Autodesk Inventor part; units mm, degrees
ref_plane "YZ Plane" through (0, 0, 0) normal (1, 0, 0) x (0, 1, 0)
ref_plane "XZ Plane" through (0, 0, 0) normal (0, 1, 0) x (-1, 0, 0)
ref_plane "XY Plane" through (0, 0, 0) normal (0, 0, 1) x (1, 0, 0)
sketch "Sketch6" plane through (0, 0, 0) normal (0, 1, 0) x (-1, 0, 0)
  line L0 (255.9, -490) -> (-255.9, -490)
  line L1 (-255.9, -490) -> (-255.9, 490)
  line L2 (-255.9, 490) -> (255.9, 490)
  line L3 (255.9, 490) -> (255.9, -490)
  line L4 (255.9, -490) -> (-255.9, 490) construction
  line L5 (-255.9, -490) -> (255.9, 490) construction
  point P0 (0, 0)
  dimension "d52" = 511.8
  dimension "d53" = 980
extrude "Plate2" add sketch "Sketch6" along normal blind 0.5
sketch "Sketch11" plane through (-255.4, 0, 490) normal (-1, 0, 0) x (0, -1, 0)
  line L0 (0, -980) -> (0, 0)
  line L1 (0, 0) -> (-10, 0)
  line L2 (-10, 0) -> (-10, -980)
  line L3 (-10, -980) -> (0, -980)
edge flange "Flange2" height 10 angle 90 thickness 0.5 bend radius 0.5 thickness toward (-1, 0, 0) relief tear relief width 0.5 relief depth 0.25 edges at (-255.9, 0.5, 0) wall of the first edge with corners at (-255.4, 0, -490) (-255.4, 0, 490) (-255.4, 10, 490) (-255.4, 10, -490)
bend "Bend3"
corner "Corner3"
sketch "Sketch12" plane through (-255.9, 9.5, 490) normal (0, 1, 0) x (-1, 0, 0)
  line L0 (0, -980) -> (0, 0)
  line L1 (0, 0) -> (-10, 0)
  line L2 (-10, 0) -> (-10, -980)
  line L3 (-10, -980) -> (0, -980)
edge flange "Flange3" height 10 angle 90 thickness 0.5 bend radius 0.5 thickness toward (0, 1, 0) relief tear relief width 0.5 relief depth 0.25 edges at (-255.4, 10, 0) wall of the first edge with corners at (-255.9, 9.5, -490) (-255.9, 9.5, 490) (-245.9, 9.5, 490) (-245.9, 9.5, -490)
bend "Bend4"
corner "Corner4"
sketch "Sketch13" plane through (255.4, 0, -490) normal (1, 0, 0) x (0, 1, 0)
  line L0 (0, 980) -> (0, 0)
  line L1 (0, 0) -> (10, 0)
  line L2 (10, 0) -> (10, 980)
  line L3 (10, 980) -> (0, 980)
edge flange "Flange4" height 10 angle 90 thickness 0.5 bend radius 0.5 thickness toward (1, 0, 0) relief tear relief width 0.5 relief depth 0.25 edges at (255.9, 0.5, 0) wall of the first edge with corners at (255.4, 0, 490) (255.4, 0, -490) (255.4, 10, -490) (255.4, 10, 490)
bend "Bend5"
corner "Corner5"
sketch "Sketch14" plane through (255.9, 9.5, -490) normal (0, 1, 0) x (-1, 0, 0)
  line L0 (0, 980) -> (0, 0)
  line L1 (0, 0) -> (10, 0)
  line L2 (10, 0) -> (10, 980)
  line L3 (10, 980) -> (0, 980)
edge flange "Flange5" height 10 angle 90 thickness 0.5 bend radius 0.5 thickness toward (0, 1, 0) relief tear relief width 0.5 relief depth 0.25 edges at (255.4, 10, 0) wall of the first edge with corners at (255.9, 9.5, 490) (255.9, 9.5, -490) (245.9, 9.5, -490) (245.9, 9.5, 490)
bend "Bend6"
corner "Corner6"
fillet "Corner Round1" radius 4 4 edges at (245.9, 9.75, -490) (-245.9, 9.75, -490) (-245.9, 9.75, 490) (245.9, 9.75, 490)
equation "\"d52\" = ЖАБРЫ_базовая_ширина - 4 * ЖАБРЫ_шаг_листов"
equation "\"d53\" = ЖАБРЫ_базовая_длина_кор_лист"
equation "\"d54\" = Thickness"
equation "\"d84\" = BendReliefWidth"
equation "\"d85\" = BendReliefDepth"
equation "\"d86\" = MinimumRemnant"
equation "\"d87\" = TransitionRadius"
equation "\"d90\" = BendRadius"
equation "\"d91\" = CornerReliefSize"
equation "\"d92\" = GapSize"
equation "\"d93\" = JacobiRadiusSize"
equation "\"d94\" = BendReliefWidth"
equation "\"d95\" = BendReliefDepth"
equation "\"d96\" = MinimumRemnant"
equation "\"d97\" = TransitionRadius"
equation "\"d100\" = BendRadius"
equation "\"d101\" = CornerReliefSize"
equation "\"d102\" = GapSize"
equation "\"d103\" = JacobiRadiusSize"
equation "\"d104\" = BendReliefWidth"
equation "\"d105\" = BendReliefDepth"
equation "\"d106\" = MinimumRemnant"
equation "\"d107\" = TransitionRadius"
equation "\"d110\" = BendRadius"
equation "\"d111\" = CornerReliefSize"
equation "\"d112\" = GapSize"
equation "\"d113\" = JacobiRadiusSize"
equation "\"d114\" = BendReliefWidth"
equation "\"d115\" = BendReliefDepth"
equation "\"d116\" = MinimumRemnant"
equation "\"d117\" = TransitionRadius"
equation "\"d120\" = BendRadius"
equation "\"d121\" = CornerReliefSize"
equation "\"d122\" = GapSize"
equation "\"d123\" = JacobiRadiusSize"
equation "\"BendRadius\" = Thickness"
equation "\"BendReliefWidth\" = Thickness"
equation "\"BendReliefDepth\" = 0.5 * Thickness"
equation "\"CornerReliefSize\" = 4 * Thickness"
equation "\"MinimumRemnant\" = 2 * Thickness"
equation "\"TransitionRadius\" = BendRadius"
equation "\"JacobiRadiusSize\" = BendRadius"
equation "\"GapSize\" = Thickness"
properties part number "MSC 808 SHEET GILLS" material "Stainless Steel"
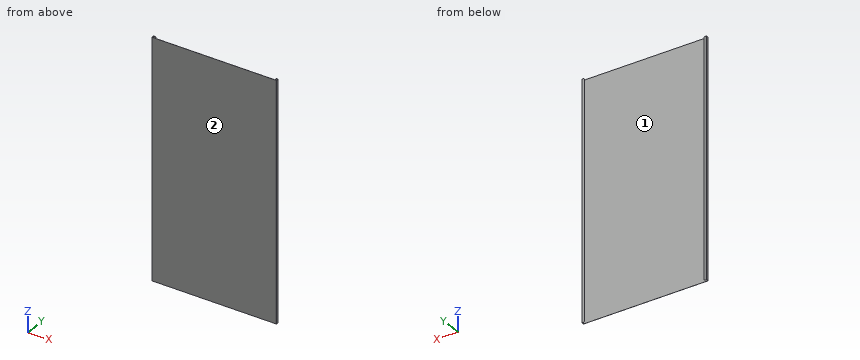
For this review, take the finished solid that the model builds, in its own axes (mm). Face numbers are marked on the shaded views. Round coordinates to 2 decimals unless told otherwise and drop trailing zeros. Loops run counter-clockwise (first coordinate to the right, second up) from the corner with the lowest first, then second, coordinate; pieces in that order, holes last.
Q1. Insertion check: pin 1 Ø0.6 at (y, z) = (9.5, -242) entering from +X; pin 2 Ø8 at (x, z) = (127.5, -306) entering from +Y. Each pin has a flat end and moves straight along its axis. Give the tip position at first contact, or say it passes through.
Result sheet:
pin 1: stops at x = 255.88
pin 2: stops at y = 0.5
Q2. To check wall thickness, follow line 1 along X through (y, z) = (4.75, -88.5); line 2 along Y through (x, z) = (187, -203.5). State the ranges of each line that lie inside material, in increasing order.
Result sheet:
line 1: x = -255.9 to -255.4, 255.4 to 255.9
line 2: y = 0 to 0.5
Q3. Add section C-C on x = -216. Write out the cut boundary in (y, z), plus the area to 3 significant figures.
Result sheet:
outline: (0, -490) - (0.5, -490) - (0.5, 490) - (0, 490) - close
area: 490 mm2
Q4. Add section A-A on y = 6.5. Write out the cut boundary in (x, z).
Result sheet:
outline: (-255.9, -490) - (-255.4, -490) - (-255.4, 490) - (-255.9, 490) - close; (255.4, -490) - (255.9, -490) - (255.9, 490) - (255.4, 490) - close
Q5. Mouldability with a two-part tool opening along X and no side actions: class the marked faces 1 and 2 as +X half, -X half, draft (parallel to the pull), parting line (faces both ways), or undercut.
Result sheet:
face 1: undercut
face 2: draft
Q6. Add section B-B on z = -211. Write out the cut boundary in (x, y).
Result sheet:
outline: (-255.9, 1) arc R1 ccw to (-254.9, 0) - (254.9, 0) arc R1 ccw to (255.9, 1) - (255.9, 9) arc R1 ccw to (254.9, 10) - (245.9, 10) - (245.9, 9.5) - (254.9, 9.5) arc R0.5 cw to (255.4, 9) - (255.4, 1) arc R0.5 cw to (254.9, 0.5) - (-254.9, 0.5) arc R0.5 cw to (-255.4, 1) - (-255.4, 9) arc R0.5 cw to (-254.9, 9.5) - (-245.9, 9.5) - (-245.9, 10) - (-254.9, 10) arc R1 ccw to (-255.9, 9) - close
